Could you check a few things on this model? Use its own coordinates, in mm. A direction names the side the tool comes from. Round coordinates to 2 decimals unless told otherwise and drop trailing zeros. Write each loop counter-clockwise with the first axis right and the second up, starting at its lowest first coordinate (ties: lowest second). Pieces come first, ordered by that corner, then holes. Notation, with made-up numbers: (37, 85.25) -> (41, 85.25) arc R15 ccw to (41, 96.25) -> close; hole circle Ø4 at (51.5, 88.25). An arc over 180 degrees is marked (long way). Answer as CSV lines item,"result". Start each with the question number.
Q1. Will these pins go through, and if not, where does the flat tip stop? pin 1 Ø1.5 at (x, z) = (-14.5, 10.5) entering from +Y; pin 2 Ø15 at (y, z) = (-4, -4.5) entering from -X; pin 3 Ø6 at (x, y) = (7, 35) entering from +Z.
Q2. Imagine slicing it at C-C on z = 0. Give the number of separate pieces and of enclosed holes in the cut face, and give its area (3 significant figures).
Q3. Imagine slicing it at D-D on z = -7. Please give me the cut outline in (x, y), and give its area (3 significant figures).
Q4. For faces 1 (the cylindrical face through (-17.54, 27.19, -1.28)), 2 (the flat face through (10.043, 10, -3)), 3 (the flat face through (-12.05, 16, 0)), which set-ups out of +Z, -Z, +X, -X, +Y, -Y let a thin tool reach every point of the face, with its end or its side?
Q5. Imagine slicing it at B-B on y = 0. Please give me the cut outline in (x, z), and give its area (3 significant figures).
Q6. If we mould it in two halves opening along X, with no side actions, what happens to faces 4 (the flat face through (17.95, 33, 0)), 5 (the flat face through (12.05, 16, 0)), 6 (the flat face through (15, 42.177, 0))? For each: pulls with the +X half, pulls with the -X half, needs draft (parallel to the pull), parting line crosses it, or undercut.
Q7. Imagine slicing it at A-A on x = -15. Please give me the cut outline in (y, z), and give its area (3 significant figures).
Q8. If I drill on line 1 (Y direction, x = -11.35, z = 0); line 2 (X direction, y = -10, z = -12); line 3 (X direction, y = 8.5, z = 8), over which ranges is the centre line in solid material (lowest first)? Write a range as [from, to].
from build123d import *

# Parameters (mm, degrees)
IZIM2_R                          = 15
IZIM2_R_2                        = 10
Y_KSEKLIK_EKSTR_ZYON1_DEPTH      = 12.05
IZIM3_R                          = 10
Y_KSEKLIK_EKSTR_ZYON2_DEPTH      = 5
IZIM4_R                          = 15
Y_KSEKLIK_EKSTR_ZYON3_DEPTH      = 5
IZIM7_R                          = 15
IZIM7_R_2                        = 10
Y_KSEKLIK_EKSTR_ZYON4_DEPTH      = 5
IZIM5_R                          = 5.907014981
Y_KSEKLIK_EKSTR_ZYON5_DEPTH      = 1
Y_KSEKLIK_EKSTR_ZYON5_DEPTH_BACK = 35
SKETCH1_W                        = 20.286238667
SKETCH1_H                        = 40.774330455
CUT_EXTRUDE1_DEPTH               = 110


with BuildPart() as part:
    # izim2 → Y_kseklik-Ekstr_zyon1 (new body, symmetric)
    with BuildSketch(Plane(origin=(0, 0, 0), x_dir=(0, 0, -1), z_dir=(1, 0, 0))):
        Circle(IZIM2_R)
        Circle(IZIM2_R_2, mode=Mode.SUBTRACT)
    extrude(amount=Y_KSEKLIK_EKSTR_ZYON1_DEPTH, both=True)

    # izim3 → Y_kseklik-Ekstr_zyon2 (add)
    with BuildSketch(Plane(origin=(12.05, 0, 0), x_dir=(0, 0, -1), z_dir=(1, 0, 0))):
        with BuildLine():
            Line((-4, 42.176870951), (4, 42.176870951))
            Line((4, 42.176870951), (17.395555059, 28.781315891))
            Line((17.395555059, 28.781315891), (22.914530919, -14.80525669))
            ThreePointArc((22.914530919, -14.80525669), (0, -26.990652818), (-22.914530919, -14.80525669))
            Line((-22.914530919, -14.80525669), (-17.395555059, 28.781315891))
            Line((-17.395555059, 28.781315891), (-4, 42.176870951))
        make_face()
        Circle(IZIM3_R, mode=Mode.SUBTRACT)
    extrude(amount=Y_KSEKLIK_EKSTR_ZYON2_DEPTH)



with BuildPart() as body_2:
    # izim4 → Y_kseklik-Ekstr_zyon3 (new body)
    with BuildSketch(Plane.ZY.offset(12.05)):
        with BuildLine():
            Line((-4, 42.176870951), (4, 42.176870951))
            Line((4, 42.176870951), (17.395555059, 28.781315891))
            Line((17.395555059, 28.781315891), (22.914530919, -14.80525669))
            ThreePointArc((22.914530919, -14.80525669), (0, -26.990652818), (-22.914530919, -14.80525669))
            Line((-22.914530919, -14.80525669), (-17.395555059, 28.781315891))
            Line((-17.395555059, 28.781315891), (-4, 42.176870951))
        make_face()
        Circle(IZIM4_R, mode=Mode.SUBTRACT)
    extrude(amount=Y_KSEKLIK_EKSTR_ZYON3_DEPTH)


with BuildPart() as part_1:
    add(part.part)

    add(body_2.part)  # Y_kseklik-Ekstr_zyon4 merges body 2
    # izim7 → Y_kseklik-Ekstr_zyon4 (add)
    with BuildSketch(Plane.ZY.offset(12.05)):
        Circle(IZIM7_R)
        Circle(IZIM7_R_2, mode=Mode.SUBTRACT)
    extrude(amount=Y_KSEKLIK_EKSTR_ZYON4_DEPTH)

    # izim5 → Y_kseklik-Ekstr_zyon5 (add, two sides)
    with BuildSketch(Plane.ZY.offset(17.05)) as y_kseklik_ekstr_zyon5_sk:
        with Locations((0, 32.957419359)):
            Circle(IZIM5_R)
    extrude(amount=Y_KSEKLIK_EKSTR_ZYON5_DEPTH)
    extrude(y_kseklik_ekstr_zyon5_sk.sketch, amount=-Y_KSEKLIK_EKSTR_ZYON5_DEPTH_BACK)

    # Sketch1 → Cut-Extrude1 (cut)
    with BuildSketch(Plane.XY.offset(68.760639517)):
        with Locations((-0.100463281, -3.811592274)):
            Rectangle(SKETCH1_W, SKETCH1_H)
    extrude(amount=-CUT_EXTRUDE1_DEPTH, mode=Mode.SUBTRACT)


solid = part_1.part
Checks:
1,pin 1,"y = 36.43"
1,pin 2,"x = -17.05"
1,pin 3,"z = 5.91"
2,separate pieces,"3"
2,enclosed holes,"0"
2,area,"837 mm^2"
3,outline,"(-17.05, -26.09) -> (-12.05, -26.09) -> (-12.05, -13.27) -> (-10.24, -13.27) -> (-10.24, -7.14) -> (-17.05, -7.14) -> close; (-17.05, 7.14) -> (-10.24, 7.14) -> (-10.24, 13.27) -> (-12.05, 13.27) -> (-12.05, 39.18) -> (-17.05, 39.18) -> close; (10.04, -13.27) -> (12.05, -13.27) -> (12.05, -26.09) -> (17.05, -26.09) -> (17.05, -7.14) -> (10.04, -7.14) -> close; (10.04, 7.14) -> (17.05, 7.14) -> (17.05, 39.18) -> (12.05, 39.18) -> (12.05, 13.27) -> (10.04, 13.27) -> close"
3,area,"557 mm^2"
4,face 1,"-X"
4,face 2,"+Z, -Z, -Y"
4,face 3,"none"
5,outline,"(-17.05, -21.04) -> (-12.05, -21.04) -> (-12.05, -15) -> (-10.24, -15) -> (-10.24, -10) -> (-17.05, -10) -> close; (-17.05, 10) -> (-10.24, 10) -> (-10.24, 15) -> (-12.05, 15) -> (-12.05, 21.04) -> (-17.05, 21.04) -> close; (10.04, -15) -> (12.05, -15) -> (12.05, -21.04) -> (17.05, -21.04) -> (17.05, -10) -> (10.04, -10) -> close; (10.04, 10) -> (17.05, 10) -> (17.05, 21.04) -> (12.05, 21.04) -> (12.05, 15) -> (10.04, 15) -> close"
5,area,"259 mm^2"
6,face 4,"pulls with the +X half"
6,face 5,"undercut"
6,face 6,"needs draft"
7,outline,"(-14.81, -22.91) -> (28.78, -17.4) -> (42.18, -4) -> (42.18, 4) -> (28.78, 17.4) -> (-14.81, 22.91) arc R27.64 ccw to start; hole circle Ø20 at (0, 0)"
7,area,"2,120 mm^2"
8,line 1,"[-15, -10], [10, 15], [27.05, 38.86]"
8,line 2,"[-17.05, -12.05], [12.05, 17.05]"
8,line 3,"[-17.05, -10.24], [10.04, 17.05]"
